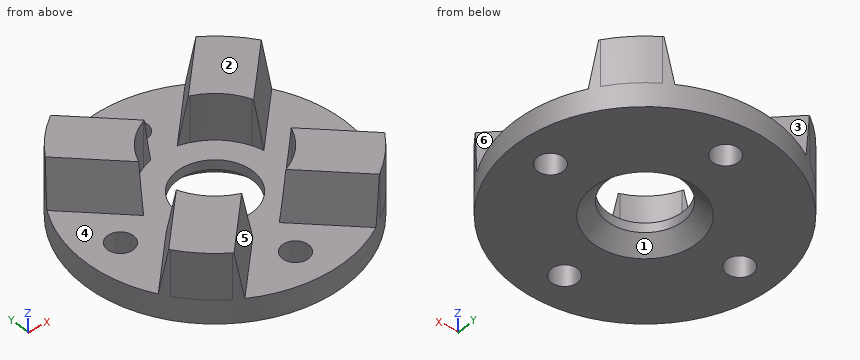
```python
from build123d import *
from build123d.topology import SkipClean

# Parameters (mm, degrees)
SZKIC1_R                    = 11
SZKIC1_R_2                  = 1.1
SZKIC1_R_3                  = 3.2
DODANIE_WYCI_GNI_CIE1_DEPTH = 2
SFAZOWANIE1_SIZE            = 1.2
DODANIE_WYCI_GNI_CIE2_DEPTH = 3.9
SZYK_KO_OWY1_COUNT          = 4


with BuildPart() as part:
    # Szkic1 → Dodanie-wyciągnięcie1 (new body)
    with BuildSketch(Plane.XY):
        Circle(SZKIC1_R)
        with Locations((0, 8)):
            Circle(SZKIC1_R_2, mode=Mode.SUBTRACT)
        with Locations((8, 0)):
            Circle(SZKIC1_R_2, mode=Mode.SUBTRACT)
        with Locations((0, -8)):
            Circle(SZKIC1_R_2, mode=Mode.SUBTRACT)
        with Locations((-8, 0)):
            Circle(SZKIC1_R_2, mode=Mode.SUBTRACT)
        Circle(SZKIC1_R_3, mode=Mode.SUBTRACT)
    extrude(amount=DODANIE_WYCI_GNI_CIE1_DEPTH)

    # Sfazowanie1
    sfazowanie1_edges = [part.edges().sort_by_distance(p)[0] for p in [
        (-3.2, 0, 0),
    ]]
    chamfer(sfazowanie1_edges, length=SFAZOWANIE1_SIZE)

    # Szkic2 → Dodanie-wyciągnięcie2 (add)
    with BuildSketch(Plane.XY.offset(2)):
        with BuildLine():
            ThreePointArc((-1.985434, -4.806043), (-3.681187, -3.672719), (-4.810603, -1.974361))
            Line((-4.810603, -1.974361), (-9.069916, -6.223876))
            ThreePointArc((-9.069916, -6.223876), (-7.787126, -7.769213), (-6.244747, -9.055558))
            Line((-6.244747, -9.055558), (-1.985434, -4.806043))
        make_face()
    dodanie_wyci_gni_cie2 = extrude(amount=DODANIE_WYCI_GNI_CIE2_DEPTH)

    # Sfazowanie2
    # the kernel refuses this chamfer: 4.537025, 0.8 mm, written as the material it adds along each edge
    with BuildSketch(Plane(origin=(-9.583198, -12.386329, 2), x_dir=(0.6905216935845088, -0.6921137853794768, -0.21013876076743532), z_dir=(0.7079205386909484, 0.7062920861085148, 0))) as sfazowanie2_piece_1_section:
        with BuildLine():
            Line((0.850504, 0), (-1.021772, -4.603832))
            Line((-1.021772, -4.603832), (-1.110486, -4.584764))
            ThreePointArc((-1.110486, -4.584764), (-0.584195, -2.286159), (-0.088714, 0.019068))
            Line((-0.088714, 0.019068), (0.019068, 0.088714))
            ThreePointArc((0.019068, 0.088714), (0.425542, 0.001348), (0.869572, 0.088714))
            Line((0.869572, 0.088714), (0.850504, 0))
        make_face()
    sfazowanie2_piece_1 = extrude(amount=15.448363, mode=Mode.PRIVATE)
    sfazowanie2_piece_1 = sfazowanie2_piece_1 & Plane(origin=(0, 0, 3.473848), x_dir=(1, 0, 0), z_dir=(0, 0, -1)) * Cylinder(11, 50, mode=Mode.PRIVATE)
    sfazowanie2_piece_1 = sfazowanie2_piece_1 - Plane(origin=(0, 0, 3.473848), x_dir=(-0.38181431028836865, -0.9242390559043788, 0), z_dir=(0, 0, -1)) * Cylinder(5.2, 50, mode=Mode.PRIVATE)
    sfazowanie2_piece_1 = split(sfazowanie2_piece_1, bisect_by=Plane(origin=(-3.895318, -7.039482, 5.9), z_dir=(0, 0, -1)), keep=Keep.TOP, mode=Mode.PRIVATE)
    add(sfazowanie2_piece_1)
    with BuildSketch(Plane(origin=(-1.472152, 1.35641, 2), x_dir=(-0.690521693584509, 0.6921137853794764, -0.21013876076743535), z_dir=(-0.7079205386909481, -0.706292086108515, 0))) as sfazowanie2_piece_2_section:
        with BuildLine():
            Line((0.850504, 0), (-1.021772, -4.603832))
            Line((-1.021772, -4.603832), (-1.110486, -4.584764))
            ThreePointArc((-1.110486, -4.584764), (-0.584195, -2.286159), (-0.088714, 0.019068))
            Line((-0.088714, 0.019068), (0.019068, 0.088714))
            ThreePointArc((0.019068, 0.088714), (0.425542, 0.001348), (0.869572, 0.088714))
            Line((0.869572, 0.088714), (0.850504, 0))
        make_face()
    sfazowanie2_piece_2 = extrude(amount=15.448363, mode=Mode.PRIVATE)
    sfazowanie2_piece_2 = sfazowanie2_piece_2 - Plane(origin=(0, 0, 3.473848), x_dir=(-0.38181431028836865, -0.9242390559043788, 0), z_dir=(0, 0, -1)) * Cylinder(5.2, 50, mode=Mode.PRIVATE)
    sfazowanie2_piece_2 = sfazowanie2_piece_2 & Plane(origin=(0, 0, 3.473848), x_dir=(1, 0, 0), z_dir=(0, 0, -1)) * Cylinder(11, 50, mode=Mode.PRIVATE)
    sfazowanie2_piece_2 = split(sfazowanie2_piece_2, bisect_by=Plane(origin=(-7.048434, -3.879096, 5.9), z_dir=(0, 0, -1)), keep=Keep.TOP, mode=Mode.PRIVATE)
    add(sfazowanie2_piece_2)

    # Szyk kołowy1: Dodanie-wyciągnięcie2 ×4 about axis
    with SkipClean():  # the faces are left unmerged after this step: merging them gives an invalid solid
        szyk_ko_owy1_axis = Axis((0, 0, 0), (0, 0, 1))
        for i in range(1, SZYK_KO_OWY1_COUNT):
            add(dodanie_wyci_gni_cie2.rotate(szyk_ko_owy1_axis, i * 360 / SZYK_KO_OWY1_COUNT))

    # Sfazowanie2 of Szyk kołowy1
    # the kernel refuses this chamfer: 4.537025, 0.8 mm, written as the material it adds along each edge
    with BuildSketch(Plane(origin=(12.386329, -9.583198, 2), x_dir=(0.6921137853794768, 0.6905216935845088, -0.21013876076743532), z_dir=(-0.7062920861085147, 0.7079205386909485, 0))) as sfazowanie2_of_szyk_ko_owy1_piece_1_section:
        with BuildLine():
            Line((0.850504, 0), (-1.021772, -4.603832))
            Line((-1.021772, -4.603832), (-1.110486, -4.584764))
            ThreePointArc((-1.110486, -4.584764), (-0.584195, -2.286159), (-0.088714, 0.019068))
            Line((-0.088714, 0.019068), (0.019068, 0.088714))
            ThreePointArc((0.019068, 0.088714), (0.425542, 0.001348), (0.869572, 0.088714))
            Line((0.869572, 0.088714), (0.850504, 0))
        make_face()
    sfazowanie2_of_szyk_ko_owy1_piece_1 = extrude(amount=15.448363, mode=Mode.PRIVATE)
    sfazowanie2_of_szyk_ko_owy1_piece_1 = sfazowanie2_of_szyk_ko_owy1_piece_1 & Plane(origin=(0, 0, 3.473848), x_dir=(1, 0, 0), z_dir=(0, 0, -1)) * Cylinder(11, 50, mode=Mode.PRIVATE)
    sfazowanie2_of_szyk_ko_owy1_piece_1 = sfazowanie2_of_szyk_ko_owy1_piece_1 - Plane(origin=(0, 0, 3.473848), x_dir=(0.9242390559043788, -0.38181431028836876, 0), z_dir=(0, 0, -1)) * Cylinder(5.2, 50, mode=Mode.PRIVATE)
    sfazowanie2_of_szyk_ko_owy1_piece_1 = split(sfazowanie2_of_szyk_ko_owy1_piece_1, bisect_by=Plane(origin=(7.039482, -3.895318, 5.9), z_dir=(0, 0, -1)), keep=Keep.TOP, mode=Mode.PRIVATE)
    add(sfazowanie2_of_szyk_ko_owy1_piece_1)
    with BuildSketch(Plane(origin=(-1.35641, -1.472152, 2), x_dir=(-0.6921137853794764, -0.690521693584509, -0.21013876076743537), z_dir=(0.7062920861085149, -0.7079205386909482, 0))) as sfazowanie2_of_szyk_ko_owy1_piece_2_section:
        with BuildLine():
            Line((0.850504, 0), (-1.021772, -4.603832))
            Line((-1.021772, -4.603832), (-1.110486, -4.584764))
            ThreePointArc((-1.110486, -4.584764), (-0.584195, -2.286159), (-0.088714, 0.019068))
            Line((-0.088714, 0.019068), (0.019068, 0.088714))
            ThreePointArc((0.019068, 0.088714), (0.425542, 0.001348), (0.869572, 0.088714))
            Line((0.869572, 0.088714), (0.850504, 0))
        make_face()
    sfazowanie2_of_szyk_ko_owy1_piece_2 = extrude(amount=15.448363, mode=Mode.PRIVATE)
    sfazowanie2_of_szyk_ko_owy1_piece_2 = sfazowanie2_of_szyk_ko_owy1_piece_2 - Plane(origin=(0, 0, 3.473848), x_dir=(0.9242390559043788, -0.38181431028836876, 0), z_dir=(0, 0, -1)) * Cylinder(5.2, 50, mode=Mode.PRIVATE)
    sfazowanie2_of_szyk_ko_owy1_piece_2 = sfazowanie2_of_szyk_ko_owy1_piece_2 & Plane(origin=(0, 0, 3.473848), x_dir=(1, 0, 0), z_dir=(0, 0, -1)) * Cylinder(11, 50, mode=Mode.PRIVATE)
    sfazowanie2_of_szyk_ko_owy1_piece_2 = split(sfazowanie2_of_szyk_ko_owy1_piece_2, bisect_by=Plane(origin=(3.879096, -7.048434, 5.9), z_dir=(0, 0, -1)), keep=Keep.TOP, mode=Mode.PRIVATE)
    add(sfazowanie2_of_szyk_ko_owy1_piece_2)
    with BuildSketch(Plane(origin=(9.583198, 12.386329, 2), x_dir=(-0.6905216935845088, 0.6921137853794768, -0.21013876076743532), z_dir=(-0.7079205386909485, -0.7062920861085147, 0))) as sfazowanie2_of_szyk_ko_owy1_piece_3_section:
        with BuildLine():
            Line((0.850504, 0), (-1.021772, -4.603832))
            Line((-1.021772, -4.603832), (-1.110486, -4.584764))
            ThreePointArc((-1.110486, -4.584764), (-0.584195, -2.286159), (-0.088714, 0.019068))
            Line((-0.088714, 0.019068), (0.019068, 0.088714))
            ThreePointArc((0.019068, 0.088714), (0.425542, 0.001348), (0.869572, 0.088714))
            Line((0.869572, 0.088714), (0.850504, 0))
        make_face()
    sfazowanie2_of_szyk_ko_owy1_piece_3 = extrude(amount=15.448363, mode=Mode.PRIVATE)
    sfazowanie2_of_szyk_ko_owy1_piece_3 = sfazowanie2_of_szyk_ko_owy1_piece_3 & Plane(origin=(0, 0, 3.473848), x_dir=(1, 0, 0), z_dir=(0, 0, -1)) * Cylinder(11, 50, mode=Mode.PRIVATE)
    sfazowanie2_of_szyk_ko_owy1_piece_3 = sfazowanie2_of_szyk_ko_owy1_piece_3 - Plane(origin=(0, 0, 3.473848), x_dir=(0.38181431028836876, 0.9242390559043788, 0), z_dir=(0, 0, -1)) * Cylinder(5.2, 50, mode=Mode.PRIVATE)
    sfazowanie2_of_szyk_ko_owy1_piece_3 = split(sfazowanie2_of_szyk_ko_owy1_piece_3, bisect_by=Plane(origin=(3.895318, 7.039482, 5.9), z_dir=(0, 0, -1)), keep=Keep.TOP, mode=Mode.PRIVATE)
    add(sfazowanie2_of_szyk_ko_owy1_piece_3)
    with BuildSketch(Plane(origin=(1.472152, -1.35641, 2), x_dir=(0.6905216935845091, -0.6921137853794765, -0.21013876076743537), z_dir=(0.7079205386909482, 0.7062920861085149, 0))) as sfazowanie2_of_szyk_ko_owy1_piece_4_section:
        with BuildLine():
            Line((0.850504, 0), (-1.021772, -4.603832))
            Line((-1.021772, -4.603832), (-1.110486, -4.584764))
            ThreePointArc((-1.110486, -4.584764), (-0.584195, -2.286159), (-0.088714, 0.019068))
            Line((-0.088714, 0.019068), (0.019068, 0.088714))
            ThreePointArc((0.019068, 0.088714), (0.425542, 0.001348), (0.869572, 0.088714))
            Line((0.869572, 0.088714), (0.850504, 0))
        make_face()
    sfazowanie2_of_szyk_ko_owy1_piece_4 = extrude(amount=15.448363, mode=Mode.PRIVATE)
    sfazowanie2_of_szyk_ko_owy1_piece_4 = sfazowanie2_of_szyk_ko_owy1_piece_4 - Plane(origin=(0, 0, 3.473848), x_dir=(0.38181431028836876, 0.9242390559043788, 0), z_dir=(0, 0, -1)) * Cylinder(5.2, 50, mode=Mode.PRIVATE)
    sfazowanie2_of_szyk_ko_owy1_piece_4 = sfazowanie2_of_szyk_ko_owy1_piece_4 & Plane(origin=(0, 0, 3.473848), x_dir=(1, 0, 0), z_dir=(0, 0, -1)) * Cylinder(11, 50, mode=Mode.PRIVATE)
    sfazowanie2_of_szyk_ko_owy1_piece_4 = split(sfazowanie2_of_szyk_ko_owy1_piece_4, bisect_by=Plane(origin=(7.048434, 3.879096, 5.9), z_dir=(0, 0, -1)), keep=Keep.TOP, mode=Mode.PRIVATE)
    add(sfazowanie2_of_szyk_ko_owy1_piece_4)
    with BuildSketch(Plane(origin=(-12.386329, 9.583198, 2), x_dir=(-0.6921137853794768, -0.6905216935845088, -0.21013876076743532), z_dir=(0.7062920861085147, -0.7079205386909485, 0))) as sfazowanie2_of_szyk_ko_owy1_piece_5_section:
        with BuildLine():
            Line((0.850504, 0), (-1.021772, -4.603832))
            Line((-1.021772, -4.603832), (-1.110486, -4.584764))
            ThreePointArc((-1.110486, -4.584764), (-0.584195, -2.286159), (-0.088714, 0.019068))
            Line((-0.088714, 0.019068), (0.019068, 0.088714))
            ThreePointArc((0.019068, 0.088714), (0.425542, 0.001348), (0.869572, 0.088714))
            Line((0.869572, 0.088714), (0.850504, 0))
        make_face()
    sfazowanie2_of_szyk_ko_owy1_piece_5 = extrude(amount=15.448363, mode=Mode.PRIVATE)
    sfazowanie2_of_szyk_ko_owy1_piece_5 = sfazowanie2_of_szyk_ko_owy1_piece_5 & Plane(origin=(0, 0, 3.473848), x_dir=(1, 0, 0), z_dir=(0, 0, -1)) * Cylinder(11, 50, mode=Mode.PRIVATE)
    sfazowanie2_of_szyk_ko_owy1_piece_5 = sfazowanie2_of_szyk_ko_owy1_piece_5 - Plane(origin=(0, 0, 3.473848), x_dir=(-0.9242390559043787, 0.3818143102883689, 0), z_dir=(0, 0, -1)) * Cylinder(5.2, 50, mode=Mode.PRIVATE)
    sfazowanie2_of_szyk_ko_owy1_piece_5 = split(sfazowanie2_of_szyk_ko_owy1_piece_5, bisect_by=Plane(origin=(-7.039482, 3.895318, 5.9), z_dir=(0, 0, -1)), keep=Keep.TOP, mode=Mode.PRIVATE)
    add(sfazowanie2_of_szyk_ko_owy1_piece_5)
    with BuildSketch(Plane(origin=(1.35641, 1.472152, 2), x_dir=(0.6921137853794764, 0.690521693584509, -0.21013876076743535), z_dir=(-0.7062920861085149, 0.7079205386909482, 0))) as sfazowanie2_of_szyk_ko_owy1_piece_6_section:
        with BuildLine():
            Line((0.850504, 0), (-1.021772, -4.603832))
            Line((-1.021772, -4.603832), (-1.110486, -4.584764))
            ThreePointArc((-1.110486, -4.584764), (-0.584195, -2.286159), (-0.088714, 0.019068))
            Line((-0.088714, 0.019068), (0.019068, 0.088714))
            ThreePointArc((0.019068, 0.088714), (0.425542, 0.001348), (0.869572, 0.088714))
            Line((0.869572, 0.088714), (0.850504, 0))
        make_face()
    sfazowanie2_of_szyk_ko_owy1_piece_6 = extrude(amount=15.448363, mode=Mode.PRIVATE)
    sfazowanie2_of_szyk_ko_owy1_piece_6 = sfazowanie2_of_szyk_ko_owy1_piece_6 - Plane(origin=(0, 0, 3.473848), x_dir=(-0.9242390559043787, 0.3818143102883689, 0), z_dir=(0, 0, -1)) * Cylinder(5.2, 50, mode=Mode.PRIVATE)
    sfazowanie2_of_szyk_ko_owy1_piece_6 = sfazowanie2_of_szyk_ko_owy1_piece_6 & Plane(origin=(0, 0, 3.473848), x_dir=(1, 0, 0), z_dir=(0, 0, -1)) * Cylinder(11, 50, mode=Mode.PRIVATE)
    sfazowanie2_of_szyk_ko_owy1_piece_6 = split(sfazowanie2_of_szyk_ko_owy1_piece_6, bisect_by=Plane(origin=(-3.879096, 7.048434, 5.9), z_dir=(0, 0, -1)), keep=Keep.TOP, mode=Mode.PRIVATE)
    add(sfazowanie2_of_szyk_ko_owy1_piece_6)


solid = part.part
```
Source: CAD feature listing. Evaluate the final solid. Frame: model axes, mm. Face numbers are marked on the shaded views. A direction names the side the tool comes from. Give positions to 0.01 mm unless a question says otherwise; leave off trailing zeros. Write each loop counter-clockwise with the first axis right and the second up, starting at its lowest first coordinate (ties: lowest second). Pieces come first, ordered by that corner, then holes.
1. Section query A-A (x = 0). Return the cut outline in (y, z), then the cut area to 3 significant figures.
2. Access query for the marked faces 4, 5 and 6. Directions: +Z, -Z, +X, -X, +Y, -Y. A direction counts if a zero-diameter tool reaches every point of the face in a straight line with its end or side. Return the directions, or none.
3. Material intervals for line 1 along Y through (x, z) = (0, 1.6); line 2 along Y through (x, z) = (0, 0.9); line 3 along Z through (x, y) = (9.5, 2.75), sorted ascending.
4. Section query C-C (z = 2.9). Count the separate pieces of the cut face and the enclosed holes in it, then the cut area to 3 significant figures.
5. Section query D-D (x = 8). Return the cut outline in (y, z), then the cut area to 3 significant figures.
6. Pull-direction query (Y, two-part tool) for the marked faces 1, 2 and 3; classes: +Y half, -Y half, draft (parallel to the pull), parting line (faces both ways), or undercut.
7. First-contact query: pin 1 (8 mm diameter, centred on x = 4.5, y = -2.5, fed in from +Z); pin 2 (2 mm diameter, centred on x = 0, y = 8, fed in from +Z); pin 3 (3 mm diameter, centred on x = -2, z = 1.5, fed in from +Y). Flat tips, straight axial feed; report the tip coordinate or a pass-through.
Output values:
1. outline: (-11, 0) - (-9.1, 0) - (-9.1, 2) - (-11, 2) - close; (-6.9, 0) - (-4.4, 0) - (-3.2, 1.2) - (-3.2, 2) - (-6.9, 2) - close; (3.2, 1.2) - (4.4, 0) - (6.9, 0) - (6.9, 2) - (3.2, 2) - close; (9.1, 0) - (11, 0) - (11, 2) - (9.1, 2) - close
1. area: 21.0 mm2
2. face 4: +Z
2. face 5: +Z, -Y
2. face 6: +Z, +X
3. line 1: y = -11 to -9.1, -6.9 to -3.2, 3.2 to 6.9, 9.1 to 11
3. line 2: y = -11 to -9.1, -6.9 to -3.5, 3.5 to 6.9, 9.1 to 11
3. line 3: z = 0 to 2
4. separate pieces: 4
4. enclosed holes: 0
4. area: 125 mm2
5. outline: (-7.55, 0) - (-1.1, 0) - (-1.1, 2) - (-4.05, 2) - (-5.03, 5.9) - (-7.55, 5.9) - close; (1.1, 0) - (7.55, 0) - (7.55, 5.9) - (5, 5.9) - (4.03, 2) - (1.1, 2) - close
5. area: 49.4 mm2
6. face 1: undercut
6. face 2: draft
6. face 3: +Y half
7. pin 1: stops at z = 5.9
7. pin 2: passes through
7. pin 3: stops at y = 10.99
